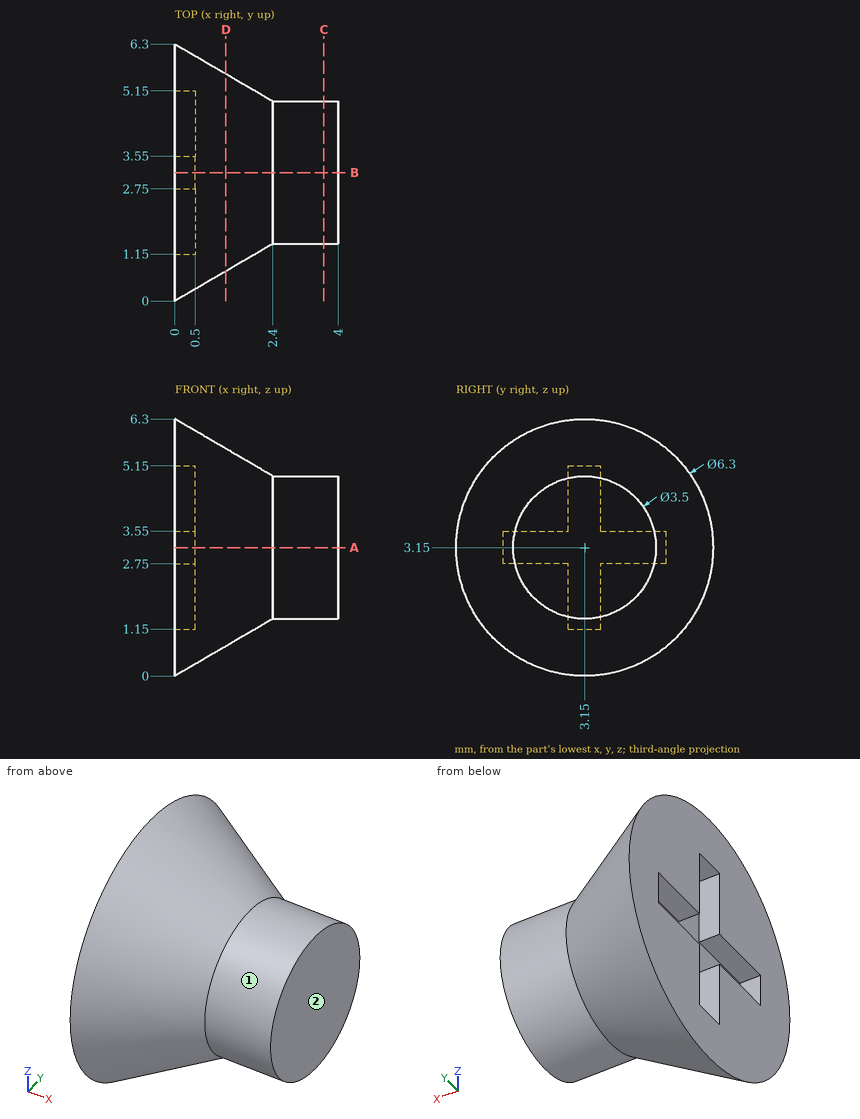
The figure shows three views and two pictorial views of one solid part (mm, origin at its lowest corner). Answer the questions. A direction names the side the tool comes from. Give positions to 0.01 mm unless a question says otherwise; leave off trailing zeros. Order: outer loops, then holes, each group sorted by start corner. A loop starts at its lowest first (then second) coordinate and runs counter-clockwise, first axis right, second up. Notation, with made-up numbers: M -14,47 L 8,47 A23 ccw 8,65 Z; hole C 50.5,86.5 d11. An arc over 180 degrees is marked long. Return JSON: item names as keys, results as strings.
Q1. Each of these flat-tipped pins is pushed along its axis until it touches: pin 1 (0.6 mm diameter, centred on x = 0, z = 4.5, fed in from +Y); pin 2 (1.5 mm diameter, centred on y = 3.5, z = 1, fed in from -X); pin 3 (1 mm diameter, centred on x = 2.5, z = 3, fed in from -Y); pin 4 (1.5 mm diameter, centred on x = 2, y = 4, fed in from -Z). Where does it stop, or does it pass through?
Answer below:
{"pin 1": "stops at y = 6.12", "pin 2": "stops at x = 0", "pin 3": "stops at y = 1.17", "pin 4": "stops at z = 0.83"}
Q2. Find section D-D, the plane x = 1.25. Write down the section's boundary in (y, z), and give its area (3 significant figures).
Answer below:
{"outline": "C 3.15,3.15 d4.84", "area": "18.4 mm^2"}
Q3. Which of the six approach directions +Z, -Z, +X, -X, +Y, -Y give full straight-line access (tool end or side, diameter ignored) to the marked faces 1 and 2?
Answer below:
{"face 1": "+X", "face 2": "+Z, -Z, +X, +Y, -Y"}
Q4. Find the intervals of material crossed by line 1 along X through (y, z) = (1.5, 3.5); line 2 along Z through (x, y) = (1.15, 4.75); line 3 along Z through (x, y) = (0.4, 4.5), in increasing order. Write a range as [from, to].
Answer below:
{"line 1": "x = [0.5, 4]", "line 2": "z = [1.26, 5.04]", "line 3": "z = [0.56, 2.75], [3.55, 5.74]"}
Q5. Find section A-A, the plane z = 3.15. Write down the section's boundary in (x, y).
Answer below:
{"outline": "M 0,0 L 2.4,1.4 L 4,1.4 L 4,4.9 L 2.4,4.9 L 0,6.3 L 0,5.15 L 0.5,5.15 L 0.5,1.15 L 0,1.15 Z"}
Q6. Find section C-C, the plane x = 3.65. Write down the section's boundary in (y, z), and give its area (3 significant figures).
Answer below:
{"outline": "C 3.15,3.15 d3.5", "area": "9.62 mm^2"}
